```python
from build123d import *

# Parameters (mm, degrees)
SKETCH1_R           = 32.7406
SKETCH1_W           = 31
SKETCH1_H           = 31
BOSS_EXTRUDE1_DEPTH = 20
SKETCH2_R           = 32.7406
SKETCH2_R_2         = 25.4
CUT_EXTRUDE1_DEPTH  = 1


with BuildPart() as part:
    # Sketch1 → Boss-Extrude1 (new body)
    with BuildSketch(Plane.XY):
        Circle(SKETCH1_R)
        Rectangle(SKETCH1_W, SKETCH1_H, mode=Mode.SUBTRACT)
    extrude(amount=BOSS_EXTRUDE1_DEPTH)

    # Sketch2 → Cut-Extrude1 (cut)
    with BuildSketch(Plane.XY.offset(20)):
        Circle(SKETCH2_R)
        Circle(SKETCH2_R_2, mode=Mode.SUBTRACT)
    extrude(amount=-CUT_EXTRUDE1_DEPTH, mode=Mode.SUBTRACT)


solid = part.part
```
For this review, take the finished solid that the model builds, in its own axes (mm). A direction names the side the tool comes from. Give positions to 0.01 mm unless a question says otherwise; leave off trailing zeros. Write each loop counter-clockwise with the first axis right and the second up, starting at its lowest first coordinate (ties: lowest second). Pieces come first, ordered by that corner, then holes.
Item 1: Machinability: for faces 1 (the face through (0, -15.5, 10)), 2 (the face through (0, -21, 0)), 3 (the face through (16.82, -19.25, 19)), which of the approach directions +Z, -Z, +X, -X, +Y, -Y give a long, thin tool a straight path to every point of the face, cutting with its end or side? Answer none if there is none.
Item 2: Take a section at D-D (y = 21.5). Give the boundary of the cut face in (x, z), and give its area (3 significant figures).
Item 3: Wall thickness on probe 1 along Y at (x, z) = (-1, 6.75); probe 2 along X at (y, z) = (-0.5, 15.25); probe 3 along Z at (x, y) = (15.5, -21): over which ranges is each line inside the solid? List them lowest first.
Item 4: The part is to be moulded in two halves that separate along X. For faces 4 (the face through (-5.506, -24.796, 19.507)), 5 (the face through (0, 15.5, 10)), 6 (the face through (0, -17, 20)), say which applies: +X half, -X half, draft (parallel to the pull), parting line (faces both ways), or undercut.
Item 5: Insertion check: P1, Ø1.5, axis at x = 14, z = 10, coming from the -Y side; P2, Ø8, axis at x = 15.5, z = 12, coming from the -Y side; P3, Ø5, axis at y = -24, z = 14, coming from the -X side. Each pin has a flat end and moves straight along its axis. Give the tip position at first contact, or say it passes through.
Item 6: Take a section at B-B (z = 11.25). Give the boundary of the cut face in (x, y).
Item 7: Take a section at A-A (x = 0). Give the boundary of the cut face in (y, z).
Established:
1. face 1: +Z, -Z
1. face 2: -Z, +X, -X, +Y, -Y
1. face 3: +Z
2. outline: (-24.69, 0) - (24.69, 0) - (24.69, 19) - (13.52, 19) - (13.52, 20) - (-13.52, 20) - (-13.52, 19) - (-24.69, 19) - close
2. area: 965 mm2
3. probe 1: y = -32.73 to -15.5, 15.5 to 32.73
3. probe 2: x = -32.74 to -15.5, 15.5 to 32.74
3. probe 3: z = 0 to 19
4. face 4: parting line
4. face 5: undercut
4. face 6: draft
5. P1: stops at y = -29.94
5. P2: stops at y = -30.65
5. P3: stops at x = -24.69
6. outline: circle Ø65.48 at (0, 0); hole (-15.5, -15.5) - (15.5, -15.5) - (15.5, 15.5) - (-15.5, 15.5) - close
7. outline: (-32.74, 0) - (-15.5, 0) - (-15.5, 20) - (-25.4, 20) - (-25.4, 19) - (-32.74, 19) - close; (15.5, 0) - (32.74, 0) - (32.74, 19) - (25.4, 19) - (25.4, 20) - (15.5, 20) - close
